```python
from build123d import *

# Parameters (mm, degrees)
SKETCH1_W           = 25.4
SKETCH1_H           = 25.4
SKETCH1_W_2         = 22.225
SKETCH1_H_2         = 22.225
BOSS_EXTRUDE1_DEPTH = 342.9
SKETCH2_R           = 2.5527
CUT_EXTRUDE1_DEPTH  = 345.073916477
SKETCH3_R           = 2.5527
CUT_EXTRUDE2_DEPTH  = 345.073916477


with BuildPart() as part:
    # Sketch1 → Boss-Extrude1 (new body)
    with BuildSketch(Plane.XY):
        Rectangle(SKETCH1_W, SKETCH1_H)
        Rectangle(SKETCH1_W_2, SKETCH1_H_2, mode=Mode.SUBTRACT)
    extrude(amount=BOSS_EXTRUDE1_DEPTH)

    # Sketch2 → Cut-Extrude1 (cut, through all)
    with BuildSketch(Plane(origin=(0, 12.7, 0), x_dir=(1, 0, 0), z_dir=(0, 1, 0))):
        Circle(SKETCH2_R)
        with Locations(Location((0, -12.7, 0), (0, 0, 270))):
            Circle(SKETCH2_R)
        with Locations(Location((0, -25.4, 0), (0, 0, 270))):
            Circle(SKETCH2_R)
        with Locations(Location((0, -38.1, 0), (0, 0, 270))):
            Circle(SKETCH2_R)
        with Locations(Location((0, -50.8, 0), (0, 0, 270))):
            Circle(SKETCH2_R)
        with Locations(Location((0, -63.5, 0), (0, 0, 270))):
            Circle(SKETCH2_R)
        with Locations(Location((0, -76.2, 0), (0, 0, 270))):
            Circle(SKETCH2_R)
        with Locations(Location((0, -88.9, 0), (0, 0, 270))):
            Circle(SKETCH2_R)
        with Locations(Location((0, -101.6, 0), (0, 0, 270))):
            Circle(SKETCH2_R)
        with Locations(Location((0, -114.3, 0), (0, 0, 270))):
            Circle(SKETCH2_R)
        with Locations(Location((0, -127, 0), (0, 0, 270))):
            Circle(SKETCH2_R)
        with Locations(Location((0, -139.7, 0), (0, 0, 270))):
            Circle(SKETCH2_R)
        with Locations(Location((0, -152.4, 0), (0, 0, 270))):
            Circle(SKETCH2_R)
        with Locations(Location((0, -165.1, 0), (0, 0, 270))):
            Circle(SKETCH2_R)
        with Locations(Location((0, -177.8, 0), (0, 0, 270))):
            Circle(SKETCH2_R)
        with Locations(Location((0, -190.5, 0), (0, 0, 270))):
            Circle(SKETCH2_R)
        with Locations(Location((0, -203.2, 0), (0, 0, 270))):
            Circle(SKETCH2_R)
        with Locations(Location((0, -215.9, 0), (0, 0, 270))):
            Circle(SKETCH2_R)
        with Locations(Location((0, -228.6, 0), (0, 0, 270))):
            Circle(SKETCH2_R)
        with Locations(Location((0, -241.3, 0), (0, 0, 270))):
            Circle(SKETCH2_R)
        with Locations(Location((0, -254, 0), (0, 0, 270))):
            Circle(SKETCH2_R)
        with Locations(Location((0, -266.7, 0), (0, 0, 270))):
            Circle(SKETCH2_R)
        with Locations(Location((0, -279.4, 0), (0, 0, 270))):
            Circle(SKETCH2_R)
        with Locations(Location((0, -292.1, 0), (0, 0, 270))):
            Circle(SKETCH2_R)
        with Locations(Location((0, -304.8, 0), (0, 0, 270))):
            Circle(SKETCH2_R)
        with Locations(Location((0, -317.5, 0), (0, 0, 270))):
            Circle(SKETCH2_R)
        with Locations(Location((0, -330.2, 0), (0, 0, 270))):
            Circle(SKETCH2_R)
        with Locations((0, -342.9)):
            Circle(SKETCH2_R)
        with Locations((0, -355.6)):
            Circle(SKETCH2_R)
        with Locations((0, -368.3)):
            Circle(SKETCH2_R)
    extrude(amount=-CUT_EXTRUDE1_DEPTH, mode=Mode.SUBTRACT)

    # Sketch3 → Cut-Extrude2 (cut, through all)
    with BuildSketch(Plane(origin=(12.7, 0, 0), x_dir=(0, 0, -1), z_dir=(1, 0, 0))):
        Circle(SKETCH3_R)
        with Locations(Location((-12.7, 0, 0), (0, 0, 90))):
            Circle(SKETCH3_R)
        with Locations(Location((-25.4, 0, 0), (0, 0, 90))):
            Circle(SKETCH3_R)
        with Locations(Location((-38.1, 0, 0), (0, 0, 90))):
            Circle(SKETCH3_R)
        with Locations(Location((-50.8, 0, 0), (0, 0, 90))):
            Circle(SKETCH3_R)
        with Locations(Location((-63.5, 0, 0), (0, 0, 90))):
            Circle(SKETCH3_R)
        with Locations(Location((-76.2, 0, 0), (0, 0, 90))):
            Circle(SKETCH3_R)
        with Locations(Location((-88.9, 0, 0), (0, 0, 90))):
            Circle(SKETCH3_R)
        with Locations(Location((-101.6, 0, 0), (0, 0, 90))):
            Circle(SKETCH3_R)
        with Locations(Location((-114.3, 0, 0), (0, 0, 90))):
            Circle(SKETCH3_R)
        with Locations(Location((-127, 0, 0), (0, 0, 90))):
            Circle(SKETCH3_R)
        with Locations(Location((-139.7, 0, 0), (0, 0, 90))):
            Circle(SKETCH3_R)
        with Locations(Location((-152.4, 0, 0), (0, 0, 90))):
            Circle(SKETCH3_R)
        with Locations(Location((-165.1, 0, 0), (0, 0, 90))):
            Circle(SKETCH3_R)
        with Locations(Location((-177.8, 0, 0), (0, 0, 90))):
            Circle(SKETCH3_R)
        with Locations(Location((-190.5, 0, 0), (0, 0, 90))):
            Circle(SKETCH3_R)
        with Locations(Location((-203.2, 0, 0), (0, 0, 90))):
            Circle(SKETCH3_R)
        with Locations(Location((-215.9, 0, 0), (0, 0, 90))):
            Circle(SKETCH3_R)
        with Locations(Location((-228.6, 0, 0), (0, 0, 90))):
            Circle(SKETCH3_R)
        with Locations(Location((-241.3, 0, 0), (0, 0, 90))):
            Circle(SKETCH3_R)
        with Locations(Location((-254, 0, 0), (0, 0, 90))):
            Circle(SKETCH3_R)
        with Locations(Location((-266.7, 0, 0), (0, 0, 90))):
            Circle(SKETCH3_R)
        with Locations(Location((-279.4, 0, 0), (0, 0, 90))):
            Circle(SKETCH3_R)
        with Locations(Location((-292.1, 0, 0), (0, 0, 90))):
            Circle(SKETCH3_R)
        with Locations(Location((-304.8, 0, 0), (0, 0, 90))):
            Circle(SKETCH3_R)
        with Locations(Location((-317.5, 0, 0), (0, 0, 90))):
            Circle(SKETCH3_R)
        with Locations(Location((-330.2, 0, 0), (0, 0, 90))):
            Circle(SKETCH3_R)
        with Locations((-342.9, 0)):
            Circle(SKETCH3_R)
        with Locations((-355.6, 0)):
            Circle(SKETCH3_R)
        with Locations((-368.3, 0)):
            Circle(SKETCH3_R)
    extrude(amount=-CUT_EXTRUDE2_DEPTH, mode=Mode.SUBTRACT)


solid = part.part
```
Model file for the job. Use its own axes, mm. A direction names the side the tool comes from. Coordinates: 2 decimals unless noted, no trailing zeros. Order: outer loops, then holes, each group sorted by start corner. A loop starts at its lowest first (then second) coordinate and runs counter-clockwise, first axis right, second up. Notation, with made-up numbers: (-2, 2.25) - (42, 2.25) arc R23 cw to (42, 10.25) - close; hole circle Ø4 at (56.5, 24). An arc over 180 degrees is marked (long way). Return JSON: item names as keys, results as strings. Group by question number.
1) Flat gauge pin, fed straight in: P1, Ø6.5, axis at x = 0, z = 50.8, coming from the +Y side. Where does the tip first touch, or does it go through?
2) Saw through at B-B, the plane z = 83. Write the cut outline in (x, y).
3) Tool access for faces 1 (the flat face through (0, -11.112, 169)), 2 (the flat face through (-11.4, -9.5, 342.9)): list every direction of +Z, -Z, +X, -X, +Y, -Y with a clear straight run to the whole face (end or side of a thin tool).
4) Mould opens along X. For faces 3 (the flat face through (9.9, 11.4, 342.9)), 4 (the flat face through (12.7, 0, 169)), 5 (the flat face through (0, 11.112, 169)) say: released by +X, released by -X, zero draft, split by the parting line, or undercut.
5) Saw through at A-A, the plane x = 8. Write the cut outline in (y, z), plus the area to 3 significant figures.
6) Probe line 1 (Y direction, x = 2.5, z = 309.5); line 2 (X direction, y = -11.9, z = 127). List the from-to ranges inside material, lowest first. Write a range as from..to.
Values found:
{
 "1": {"P1": "stops at y = 12.7"},
 "2": {"outline": "(-12.7, -12.7) - (12.7, -12.7) - (12.7, 12.7) - (-12.7, 12.7) - close; hole (-11.11, -11.11) - (11.11, -11.11) - (11.11, 11.11) - (-11.11, 11.11) - close"},
 "3": {"face 1": "+Z, -Z", "face 2": "+Z, +X, -X, +Y, -Y"},
 "4": {"face 3": "zero draft", "face 4": "released by +X", "face 5": "undercut"},
 "5": {"outline": "(-12.7, 0) - (-11.11, 0) - (-11.11, 342.9) - (-12.7, 342.9) - close; (11.11, 0) - (12.7, 0) - (12.7, 342.9) - (11.11, 342.9) - close", "area": "1,090 mm²"},
 "6": {"line 1": "y = -12.7..-11.11, 11.11..12.7", "line 2": "x = -12.7..-2.55, 2.55..12.7"}
}
